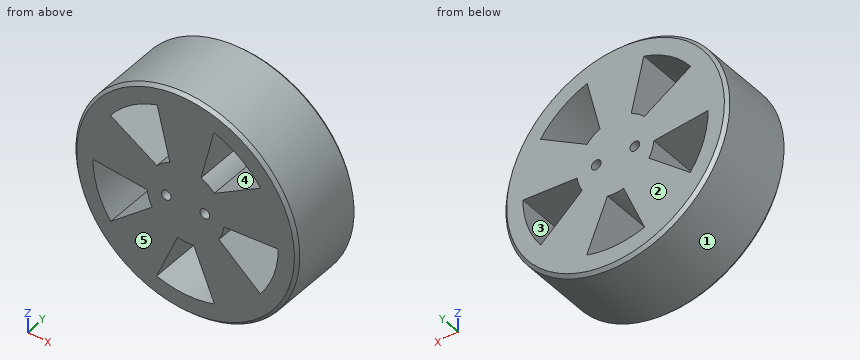
```python
from build123d import *

# Parameters (mm, degrees)
SKETCH2_R               = 73.7235
BOSS_EXTRUDE1_DEPTH     = 50.8
CHAMFER1_SIZE           = 2.032
CUT_EXTRUDE1_DEPTH      = 116.978225993
CUT_EXTRUDE1_DEPTH_BACK = 116.978225993
SKETCH3_R               = 3.175
CUT_EXTRUDE2_DEPTH      = 116.978225993
CUT_EXTRUDE2_DEPTH_BACK = 116.978225993


with BuildPart() as part:
    # Sketch2 → Boss-Extrude1 (new body)
    with BuildSketch(Plane(origin=(0, 0, 0), x_dir=(1, 0, 0), z_dir=(0, 1, 0))):
        with Locations(Location((0, 0, 0), (0, 0, 270))):
            Circle(SKETCH2_R)
    extrude(amount=BOSS_EXTRUDE1_DEPTH)

    # Chamfer1
    chamfer1_edges = [part.edges().sort_by_distance(p)[0] for p in [
        (0, 0, -73.7235),
        (0, 50.8, -73.7235),
    ]]
    chamfer(chamfer1_edges, length=CHAMFER1_SIZE)

    # Sketch3 → Cut-Extrude1 (cut, two sides: drawn at the far end of the back side and taken through both)
    with BuildSketch(Plane(origin=(0, 50.8, 0), x_dir=(1, 0, 0), z_dir=(0, 1, 0)).offset(-CUT_EXTRUDE1_DEPTH_BACK)):
        with Locations(Location((-12.7, 0, 0), (0, 0, 270))):
            Circle(SKETCH3_R)
        with Locations(Location((12.7, 0, 0), (0, 0, 270))):
            Circle(SKETCH3_R)
    extrude(amount=CUT_EXTRUDE1_DEPTH + CUT_EXTRUDE1_DEPTH_BACK, mode=Mode.SUBTRACT)

    # Sketch4 → Cut-Extrude2 (cut, two sides: drawn at the far end of the back side and taken through both)
    with BuildSketch(Plane(origin=(0, 50.8, 0), x_dir=(1, 0, 0), z_dir=(0, 1, 0)).offset(-CUT_EXTRUDE2_DEPTH_BACK)):
        with BuildLine():
            Line((-5.323781477, 24.835807834), (-19.05, 57.973830754))
            ThreePointArc((-19.05, 57.973830754), (0, 61.0235), (19.05, 57.973830754))
            Line((19.05, 57.973830754), (5.323781477, 24.835807834))
            ThreePointArc((5.323781477, 24.835807834), (0, 25.4), (-5.323781477, 24.835807834))
        make_face()
        with BuildLine():
            Line((21.975117928, 12.737903755), (49.24961577, 36.032525567))
            ThreePointArc((49.24961577, 36.032525567), (58.036797322, 18.857298556), (61.023163256, -0.202727704))
            Line((61.023163256, -0.202727704), (25.265395829, 2.611469625))
            ThreePointArc((25.265395829, 2.611469625), (24.156835514, 7.849031657), (21.975117928, 12.737903755))
        make_face()
        with BuildLine():
            Line((18.905151263, -16.963350369), (49.487936479, -35.704505253))
            ThreePointArc((49.487936479, -35.704505253), (35.868713343, -49.369048556), (18.664388993, -58.099123365))
            Line((18.664388993, -58.099123365), (10.291091885, -23.221830845))
            ThreePointArc((10.291091885, -23.221830845), (14.929745408, -20.549031657), (18.905151263, -16.963350369))
        make_face()
        with BuildLine():
            Line((-10.291091885, -23.221830845), (-18.664388993, -58.099123365))
            ThreePointArc((-18.664388993, -58.099123365), (-35.868713343, -49.369048556), (-49.487936479, -35.704505253))
            Line((-49.487936479, -35.704505253), (-18.905151263, -16.963350369))
            ThreePointArc((-18.905151263, -16.963350369), (-14.929745408, -20.549031657), (-10.291091885, -23.221830845))
        make_face()
        with BuildLine():
            Line((-25.265395829, 2.611469625), (-61.023163256, -0.202727704))
            ThreePointArc((-61.023163256, -0.202727704), (-58.036797322, 18.857298556), (-49.24961577, 36.032525567))
            Line((-49.24961577, 36.032525567), (-21.975117928, 12.737903755))
            ThreePointArc((-21.975117928, 12.737903755), (-24.156835514, 7.849031657), (-25.265395829, 2.611469625))
        make_face()
    extrude(amount=CUT_EXTRUDE2_DEPTH + CUT_EXTRUDE2_DEPTH_BACK, mode=Mode.SUBTRACT)


solid = part.part
```
Input: part model. Units: mm. Frame: model coordinates. Face numbers are marked on the shaded views. A direction names the side the tool comes from. Give positions to 0.01 mm unless a question says otherwise; leave off trailing zeros. Order: outer loops, then holes, each group sorted by start corner. A loop starts at its lowest first (then second) coordinate and runs counter-clockwise, first axis right, second up.
1. Reachability of the marked faces 4 and 5 from +Z, -Z, +X, -X, +Y, -Y: full face, straight path, thin tool, end or side. Return the list, or none.
Derived:
face 4: +Y, -Y
face 5: +Z, -Z, +X, -X, -Y
2. Mould query, pull axis Z, two halves, no side actions, for the marked faces 1, 2 and 3. Classes: released by +Z, released by -Z, zero draft, split by the parting line, or undercut.
Derived:
face 1: split by the parting line
face 2: zero draft
face 3: undercut
3. Material intervals for L1, parallel to X at y = 14.5, z = 0.5; L2, parallel to Z at x = 38.5, y = 21; L3, parallel to X at y = 32, z = 22, sorted ascending.
Derived:
L1: x = -73.72 to -15.84, -9.56 to 9.56, 15.84 to 73.72
L2: z = -62.87 to -26.85, -1.57 to 28.97, 47.35 to 62.87
L3: x = -70.36 to -27.12, -12.69 to 12.69, 27.12 to 70.36
4. Section A-A on x = 0. Return the cut outline in (y, z), and give its area (3 significant figures).
Derived:
outline: (0, -71.69) - (2.03, -73.72) - (48.77, -73.72) - (50.8, -71.69) - (50.8, -61.02) - (0, -61.02) - close; (0, -25.4) - (50.8, -25.4) - (50.8, 71.69) - (48.77, 73.72) - (2.03, 73.72) - (0, 71.69) - close
area: 5,670 mm2
5. Section B-B on y = 20.5. Give the number of separate pieces and of enclosed holes in the cut face, and give its area (3 significant figures).
Derived:
separate pieces: 1
enclosed holes: 7
area: 12,600 mm2
6. Pin query (flat end, axial travel): pin 1 (12 mm diameter, centred on x = 53.5, y = 21.5, fed in from -Z); pin 2 (2 mm diameter, centred on x = -38.5, z = -24.5, fed in from -Y); pin 3 (8.5 mm diameter, centred on x = 12.7, z = 0, fed in from -Y); pin 4 (4 mm diameter, centred on x = -40, y = 40.5, fed in from -Z). Return the tip coordinate at first contact, or that it passes through.
Derived:
pin 1: stops at z = -56.38
pin 2: passes through
pin 3: stops at y = 0
pin 4: stops at z = -63.18
